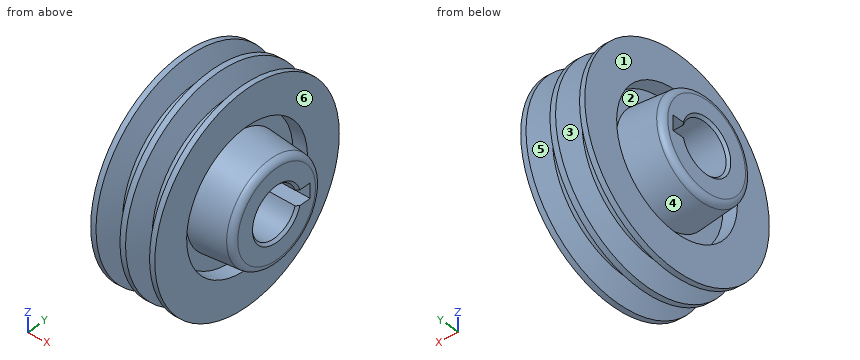
```python
from build123d import *

# Parameters (mm, degrees)
PATTERN_LINEAR_951_COUNT = 2
PATTERN_LINEAR_951_PITCH = 12
CHAMFER_1_SIZE           = 1
SKETCH_4_W               = 6
SKETCH_4_H               = 5.760607938
CUT_EXTRUDE_1_DEPTH      = 78.640195775
FILLET_2_R               = 2.5


with BuildPart() as part:
    # 草图1 → 旋转1 (revolve)
    with BuildSketch(Plane.XY, mode=Mode.PRIVATE) as revolve_1_sk:
        Polygon((-12, 10), (-12, 20), (5.5, 21.531051612), (5.5, 27.018812351), (0, 27.5), (0, 42), (26, 42), (26, 27.5), (20.5, 27.018812351), (20.5, 21.531051612), (38, 20), (38, 10), align=None)
    revolve(revolve_1_sk.sketch.rotate(Axis((0, 0, 0), (1, 0, 0)), 90), axis=Axis((0, 0, 0), (1, 0, 0)))

    # 草图2 → 切除-旋转1 (revolve, cut)
    with BuildSketch(Plane.XY, mode=Mode.PRIVATE) as cut_revolve_1_sk:
        Polygon((9.10988523, 33), (11.861461363, 42), (2.138538637, 42), (4.89011477, 33), align=None)
    cut_revolve_1 = revolve(cut_revolve_1_sk.sketch.rotate(Axis((0, 0, 0), (1, 0, 0)), 90), axis=Axis((0, 0, 0), (1, 0, 0)), mode=Mode.SUBTRACT)

    # Pattern Linear 951: 切除-旋转1 ×2
    with Locations(*[(i * PATTERN_LINEAR_951_PITCH, 0, 0) for i in range(1, PATTERN_LINEAR_951_COUNT)]):
        add(cut_revolve_1, mode=Mode.SUBTRACT)

    # 倒角1
    chamfer_1_edges = [part.edges().sort_by_distance(p)[0] for p in [
        (-12, 0, -10),
        (38, 0, -10),
    ]]
    chamfer(chamfer_1_edges, length=CHAMFER_1_SIZE)

    # 草图4 → 切除-拉伸1 (cut, through all)
    with BuildSketch(Plane.ZY.offset(12)):
        with Locations((0, 12.419695983)):
            Rectangle(SKETCH_4_W, SKETCH_4_H)
    extrude(amount=-CUT_EXTRUDE_1_DEPTH, mode=Mode.SUBTRACT)

    # 圆角2
    fillet_2_edges = [part.edges().sort_by_distance(p)[0] for p in [
        (-12, 0, -20),
        (38, 0, -20),
    ]]
    fillet(fillet_2_edges, radius=FILLET_2_R)


solid = part.part
```
Geometry: final body of the model. Coordinates: model frame, mm. Face numbers are marked on the shaded views. A direction names the side the tool comes from. Round coordinates to 2 decimals unless told otherwise and drop trailing zeros. Order: outer loops, then holes, each group sorted by start corner. A loop starts at its lowest first (then second) coordinate and runs counter-clockwise, first axis right, second up. Notation, with made-up numbers: M -0.75,2 L 43.25,2 A32 cw 43.25,34 Z; hole C 71,-38.5 d11. An arc over 180 degrees is marked long. Use one line per item in the form item = value. Start each with the question number.
Q1. Mould query, pull axis Y, two halves, no side actions, for the marked faces 1, 2 and 3. Classes: +Y half, -Y half, draft (parallel to the pull), parting line (faces both ways), or undercut.
Q2. Cut plane B-B (x = 19). Return loops of the section in (y, z).
Q3. Material intervals for line 1 (X direction, y = -32, z = 20.5); line 2 (X direction, y = 15.5, z = 31); line 3 (X direction, y = 4, z = 31.5), sorted ascending. Write a range as [from, to].
Q4. Pin query (flat end, axial travel): pin 1 Ø12 at (y, z) = (13.5, 31.5) entering from -X; pin 2 Ø6 at (x, z) = (31.5, -15.5) entering from +Y; pin 3 Ø3 at (x, z) = (12, -1) entering from -Y. Return the tip coordinate at first contact, or that it passes through.
Q5. Access query for the marked faces 4, 5 and 6. Directions: +Z, -Z, +X, -X, +Y, -Y. A direction counts if a zero-diameter tool reaches every point of the face in a straight line with its end or side. Return the directions, or none.
Q6. Cut plane A-A (x = 34). Return loops of the section in (y, z).
Geometry results:
q1.face_1 = draft
q1.face_2 = undercut
q1.face_3 = parting line
q2.outline = C 0,0 d66; hole M 9.54,-3 L 15.3,-3 L 15.3,3 L 9.54,3 A10 ccw long Z
q3.line_1 = [0, 3.36], [10.64, 15.36], [22.64, 26]
q3.line_2 = [0, 4.38], [9.62, 16.38], [21.62, 26]
q3.line_3 = [0, 26]
q4.pin_1 = 0
q4.pin_2 = 16.36
q4.pin_3 = -42
q5.face_4 = -X
q5.face_5 = none
q5.face_6 = +X
q6.outline = C 0,0 d40.7; hole M 9.54,-3 L 15.3,-3 L 15.3,3 L 9.54,3 A10 ccw long Z
